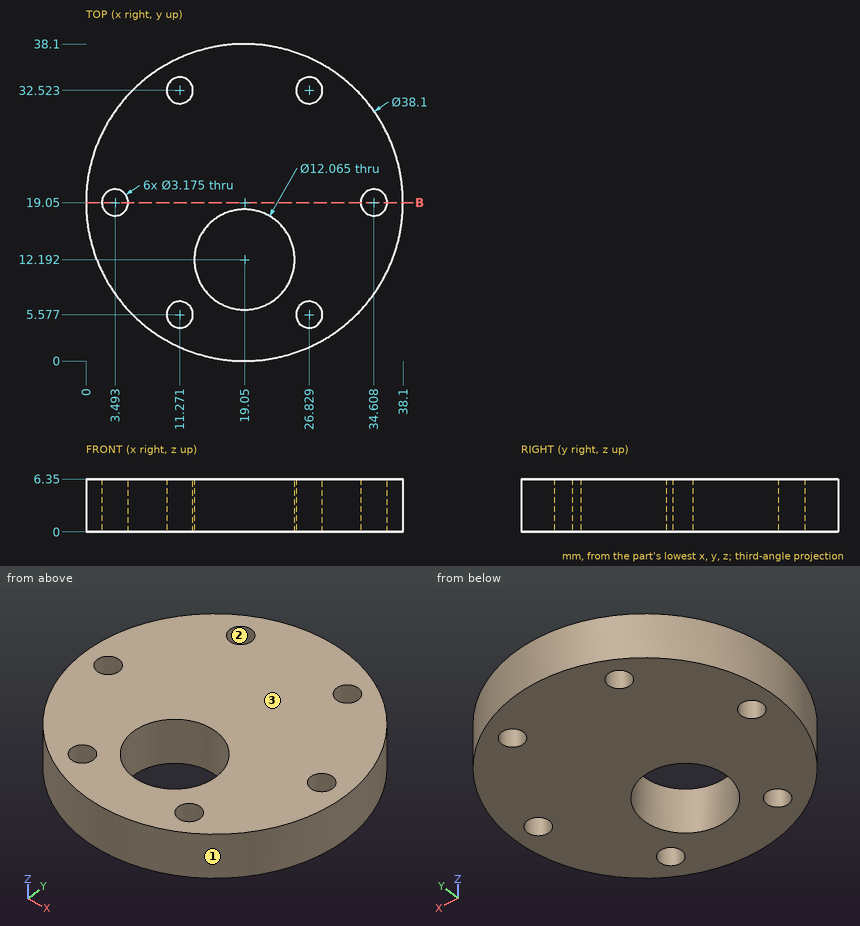
Study the drawing (mm; zero at the part's minimum x, y, z) and answer. Round coordinates to 2 decimals unless told otherwise and drop trailing zeros.
1) A cutting plane is placed at B-B on y = 19.05. Give the number of separate pieces and of enclosed holes in the cut face, and give its area (3 significant figures).
2) Determine the mould class of the marked faces 1, 2 and 3 for opening direction X: pulls with the +X half, pulls with the -X half, needs draft (parallel to the pull), parting line crosses it, or undercut.
3) Flat-ended cylindrical pins translate along their axes: P1, Ø11, axis at x = 19.05, y = 12.192, coming from the +Z side; P2, Ø3, axis at x = 18.5, z = 4, coming from the +Y side; P3, Ø2, axis at y = 20.5, z = 5, coming from the +X side (1 decimal); P4, Ø1, axis at x = 31, z = 5.5, coming from the +Y side (1 decimal). Find the tip coordinate at first contact, or state that the pin passes through.
4) Consider probe 1 along Y at (x, z) = (26, 5.25) (1 decimal); probe 2 along X at (y, z) = (20, 2) (1 decimal); probe 3 along Y at (x, z) = (32, 2). Determine where each line is inside the solid, lowest interval first.
Entries:
1. separate pieces: 3
1. enclosed holes: 0
1. area: 202 mm2
2. face 1: parting line crosses it
2. face 2: undercut
2. face 3: needs draft
3. P1: passes through
3. P2: stops at y = 38.1
3. P3: stops at x = 38.1
3. P4: stops at y = 34.3
4. probe 1: y = 1.3 to 4.2, 6.9 to 31.2, 33.9 to 36.8
4. probe 2: x = 0 to 2.2, 4.8 to 33.3, 35.9 to 38.1
4. probe 3: y = 5.08 to 33.02
